from build123d import *

# Parameters (mm, degrees)
SKETCH1_R           = 15
SKETCH1_R_2         = 13.462
BOSS_EXTRUDE1_DEPTH = 15
SKETCH4_R           = 14.2875
SKETCH4_R_2         = 13.462
SKETCH4_R_3         = 13.0429
BOSS_EXTRUDE5_DEPTH = 650
SKETCH1_4_R         = 15.875
SKETCH1_4_R_2       = 15
SKETCH1_4_R_3       = 13.462
BOSS_EXTRUDE6_DEPTH = 2


with BuildPart() as part:
    # Sketch1 → Boss-Extrude1 (new body)
    with BuildSketch(Plane(origin=(0, 0, 0), x_dir=(1, 0, 0), z_dir=(0, 1, 0))):
        with Locations(Location((0, 0, 0), (0, 0, 270))):
            Circle(SKETCH1_R)
        with Locations(Location((0, 0, 0), (0, 0, 270))):
            Circle(SKETCH1_R_2, mode=Mode.SUBTRACT)
    extrude(amount=BOSS_EXTRUDE1_DEPTH)

    # Sketch4 → Boss-Extrude5 (add)
    with BuildSketch(Plane(origin=(0, 15, 0), x_dir=(1, 0, 0), z_dir=(0, 1, 0))):
        with Locations(Location((0, 0, 0), (0, 0, 270))):
            Circle(SKETCH4_R)
        with Locations(Location((0, 0, 0), (0, 0, 270))):
            Circle(SKETCH4_R_2, mode=Mode.SUBTRACT)
        with Locations(Location((0, 0, 0), (0, 0, 270))):
            Circle(SKETCH4_R_2)
        with Locations(Location((0, 0, 0), (0, 0, 270))):
            Circle(SKETCH4_R_3, mode=Mode.SUBTRACT)
    extrude(amount=BOSS_EXTRUDE5_DEPTH)

    # Sketch1_4 → Boss-Extrude6 (add)
    with BuildSketch(Plane(origin=(0, 0, 0), x_dir=(1, 0, 0), z_dir=(0, 1, 0))):
        with Locations(Location((0, 0, 0), (0, 0, 270))):
            Circle(SKETCH1_4_R)
        with Locations(Location((0, 0, 0), (0, 0, 270))):
            Circle(SKETCH1_4_R_2, mode=Mode.SUBTRACT)
        with Locations(Location((0, 0, 0), (0, 0, 270))):
            Circle(SKETCH1_4_R_2)
        with Locations(Location((0, 0, 0), (0, 0, 270))):
            Circle(SKETCH1_4_R_3, mode=Mode.SUBTRACT)
    extrude(amount=-BOSS_EXTRUDE6_DEPTH)


solid = part.part
Could you check a few things on this model? Use its own coordinates, in mm. A direction names the side the tool comes from. Coordinates: 2 decimals unless noted, no trailing zeros. Order: outer loops, then holes, each group sorted by start corner. A loop starts at its lowest first (then second) coordinate and runs counter-clockwise, first axis right, second up. Notation, with made-up numbers: (-22, 72) -> (35, 72) arc R22 cw to (35, 100) -> close; hole circle Ø8 at (69, -37). An arc over 180 degrees is marked (long way). One line per item, written item: value. Start each with the question number.
1) We'd pull the mould along Z, two halves only. Please class faces 3 (the cylindrical face through (-7.94, 335.45, -10.35)), 4 (the cylindrical face through (0.628, 335.45, -14.274)), 5 (the flat face through (-12, 665, 6)): +Z half, -Z half, draft (parallel to the pull), parting line (faces both ways), or undercut.
2) I'm going to push flat-ended pins straight in: pin 1 (10 mm diameter, centred on y = 364, z = 6.5, fed in from +X); pin 2 (10 mm diameter, centred on y = 579.5, z = 12, fed in from +X); pin 3 (16 mm diameter, centred on x = 0, z = 0, fed in from -Y); pin 4 (12 mm diameter, centred on y = 351, z = 9, fed in from -X). Where does each tip first touch, or does it pass through?
3) Imagine slicing it at A-A on z = 0. List the corners of the cut face in (x, y) for me (1 decimal), plus the area to 3 significant figures.
4) Imagine slicing it at B-B on x = 0. List the corners of the cut face in (y, z) for me (1 decimal).
5) Which directions (+Z, -Z, +X, -X, +Y, -Y) give clear straight access to the entire face, cutting with the end or side of a thin tool? Please do faces 1 (the flat face through (-6, 0, 14)), 2 (the flat face through (-12, -2, -7)).
6) If I drill on L1, parallel to X at y = 10.5, z = 0; L2, parallel to X at y = 454.5, z = 0; L3, parallel to Z at x = -1.5, y = 415.5, over which ranges is the centre line in solid material (lowest first)? Write a range as [from, to].
7) Imagine slicing it at C-C on y = 139. List the corners of the cut face in (x, z) for me (1 decimal), plus the area to 3 significant figures.
Answer list:
1. face 3: undercut
1. face 4: parting line
1. face 5: draft
2. pin 1: stops at x = 14.21
2. pin 2: stops at x = 12.46
2. pin 3: passes through
2. pin 4: stops at x = -13.97
3. outline: (-15.9, -2) -> (-13.5, -2) -> (-13.5, 15) -> (-13, 15) -> (-13, 665) -> (-14.3, 665) -> (-14.3, 15) -> (-15, 15) -> (-15, 0) -> (-15.9, 0) -> close; (13, 15) -> (13.5, 15) -> (13.5, -2) -> (15.9, -2) -> (15.9, 0) -> (15, 0) -> (15, 15) -> (14.3, 15) -> (14.3, 665) -> (13, 665) -> close
3. area: 1,670 mm2
4. outline: (-2, -15.9) -> (0, -15.9) -> (0, -15) -> (15, -15) -> (15, -14.3) -> (665, -14.3) -> (665, -13) -> (15, -13) -> (15, -13.5) -> (-2, -13.5) -> close; (-2, 13.5) -> (15, 13.5) -> (15, 13) -> (665, 13) -> (665, 14.3) -> (15, 14.3) -> (15, 15) -> (0, 15) -> (0, 15.9) -> (-2, 15.9) -> close
5. face 1: +Y
5. face 2: +Z, -Z, +X, -X, -Y
6. L1: x = [-15, -13.46], [13.46, 15]
6. L2: x = [-14.29, -13.04], [13.04, 14.29]
6. L3: z = [-14.21, -12.96], [12.96, 14.21]
7. outline: circle Ø28.6 at (0, 0); hole circle Ø26.1 at (0, 0)
7. area: 107 mm2
